Autodesk Fusion 360 part; units mm, degrees
sketch "Sketch1" plane through (0, 0, 0) normal (0, 0, 1) x (1, 0, 0)
  circle A0 centre (0, 0) radius 2.4955
  dimension "d1" = 4.991
extrude "Extrude1" add sketch "Sketch1" along normal blind 250
thread "Thread1"

Autodesk Fusion 360 part; units mm, degrees
sketch "Sketch1" plane through (0, 0, 0) normal (0, 0, 1) x (1, 0, 0)
  circle A0 centre (10, 10) radius 2.4955
  circle A1 centre (10, 10) radius 5
  dimension "d1" = 4.991
  dimension "d2" = 10
extrude "Extrude1" add sketch "Sketch1" along normal blind 10

Autodesk Fusion 360 part; units mm, degrees
sketch "Sketch1" plane through (0, 0, 0) normal (0, 0, 1) x (1, 0, 0)
  line L0 (0, 0) -> (350, 0)
  line L1 (350, 0) -> (350, 350)
  line L2 (350, 350) -> (0, 350)
  line L3 (0, 350) -> (0, 0)
  line L4 (-10, 0) -> (-10, -10)
  line L5 (-10, -10) -> (360, -10)
  line L6 (360, -10) -> (360, 360)
  line L7 (360, 360) -> (-10, 360)
  line L8 (-10, 360) -> (-10, -10)
  dimension "d1" = 350
  dimension "d2" = 350
  dimension "d3" = 10
  dimension "d4" = 370
  dimension "d5" = 370
extrude "Extrude1" add sketch "Sketch1" along normal blind 75
sketch "Sketch2" plane through (0, 0, 0) normal (0, 0, 1) x (1, 0, 0)
  line L0 (0, 350) -> (350, 350)
  line L1 (350, 350) -> (350, 0)
  line L2 (350, 0) -> (0, 0)
  line L3 (0, 0) -> (0, 350)
extrude "Extrude2" add sketch "Sketch2" along normal blind 5

Autodesk Fusion 360 part; units mm, degrees
sketch "Sketch1" plane through (0, 0, 0) normal (0, 0, 1) x (1, 0, 0)
  line L0 (0, 0) -> (420, 0)
  line L1 (420, 0) -> (420, 420)
  line L2 (420, 420) -> (0, 420)
  line L3 (0, 420) -> (0, 0)
  dimension "d1" = 420
  dimension "d2" = 420
extrude "Extrude1" add sketch "Sketch1" along normal blind 20
sketch "Sketch2" plane through (0, 0, 20) normal (0, 0, 1) x (-1, 0, 0)
  line L0 (0, -420) -> (0, 0)
  line L1 (0, 0) -> (-420, 0)
  line L2 (-420, 0) -> (-420, -420)
  line L3 (-420, -420) -> (0, -420)
  circle A0 centre (-410, -410) radius 4
  circle A1 centre (-10, -410) radius 4
  circle A2 centre (-410, -10) radius 4
  circle A3 centre (-10, -10) radius 4
  dimension "d7" = 400
  dimension "d8" = 8
  dimension "d9" = 8
  dimension "d10" = 400
  dimension "d11" = 400
  dimension "d12" = 8
  dimension "d13" = 8
extrude "Extrude2" cut sketch "Sketch2" against normal blind 100 contours A0 | A1 | A2 | A3
extrude "Extrude3" cut 1 faces at (144.2065, 144.341, 20) along direction (0, 0, -1) blind 10

Autodesk Fusion 360 part; units mm, degrees
sketch "Sketch1" plane through (0, 0, 0) normal (0, 0, 1) x (1, 0, 0)
  line L0 (10, 10) -> (310, 10)
  line L1 (310, 10) -> (310, 60)
  line L2 (310, 60) -> (10, 60)
  line L3 (10, 60) -> (10, 10)
  dimension "d1" = 300
  dimension "d2" = 50
extrude "Extrude1" add sketch "Sketch1" along normal blind 20
Geometry check sheet. Reference: the model listing, model coordinates, mm. A direction names the side the tool comes from. Coordinates: 2 decimals unless noted, no trailing zeros. Order: outer loops, then holes, each group sorted by start corner. A loop starts at its lowest first (then second) coordinate and runs counter-clockwise, first axis right, second up. Notation, with made-up numbers: (9.25, 3) - (68.25, 3) arc R17 cw to (68.25, 32) - close; hole circle Ø5 at (60, 51). An arc over 180 degrees is marked (long way). Answer as a JSON object with one key per item and string values. Group by question number.
Item 1: Scan lines: probe 1 along X at (y, z) = (410, 22.65); probe 2 along Z at (x, y) = (101.5, 382.5). Record each from-to range of solid material in increasing order.
Item 2: Sectioned sample at C-C, the plane y = 348. Record the cut outline in (x, z), and give its area (3 significant figures).
Item 3: Depth check by flat-ended pin: pin 1 Ø8 at (x, y) = (203, 239) entering from -Z; pin 2 Ø15 at (y, z) = (26.5, 119) entering from -X; pin 3 Ø10 at (x, z) = (170.5, 48.5) entering from -Y. Enter the tip coordinate at first touch or a pass-through.
Item 4: Sectioned sample at B-B, the plane z = 73. Record the cut outline in (x, y).
Item 5: Tool access check on faces 1 (the face through (162, 60, 10)), 2 (the face through (162, 60, 136)), 3 (the face through (310, 35, 10)), 4 (the face through (158, 35, 0)), 5 (the face through (310, 35, 136)). Record the directions out of +Z, -Z, +X, -X, +Y, -Y that give a thin tool (end or side, any length) a straight path to the whole face; none if there is none.
Item 6: Sectioned sample at A-A, the plane x = 77.5. Record the cut outline in (y, z), and give its area (4 significant figures).
Resolved:
{
 "1": {"probe 1": "0 to 6, 14 to 406, 414 to 420", "probe 2": "20 to 25"},
 "2": {"outline": "(0, 20) - (420, 20) - (420, 25) - (0, 25) - close", "area": "2,100 mm^2"},
 "3": {"pin 1": "z = 20", "pin 2": "x = 10", "pin 3": "y = 10"},
 "4": {"outline": "(10, 10) - (310, 10) - (310, 60) - (10, 60) - close"},
 "5": {"face 1": "-Z, +X, -X, +Y", "face 2": "+Z, +X, -X, +Y", "face 3": "-Z, +X, +Y, -Y", "face 4": "-Z, +X, -X, +Y, -Y", "face 5": "+Z, +X, +Y, -Y"},
 "6": {"outline": "(0, 20) - (10, 20) - (10, 0) - (60, 0) - (60, 20) - (420, 20) - (420, 25) - (60, 25) - (60, 250) - (10, 250) - (10, 25) - (0, 25) - close", "area": "14,350 mm^2"}
}
